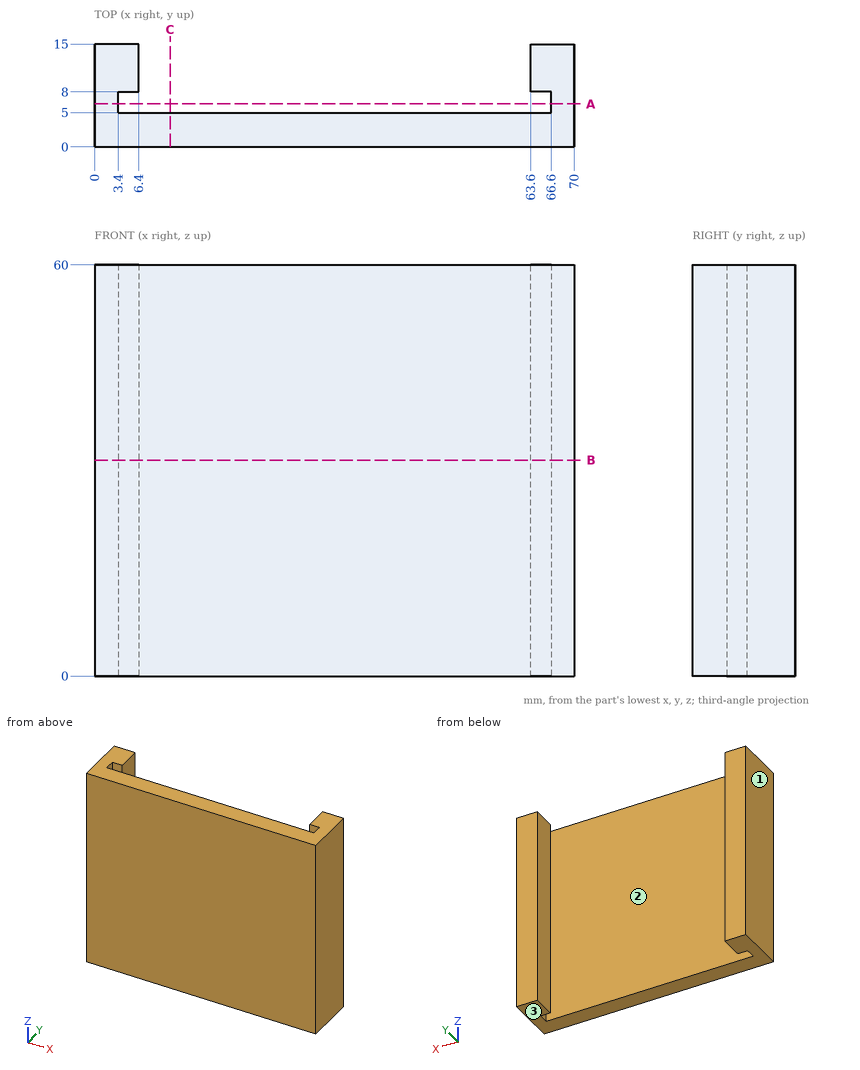
Geometry: see drawing. Coordinates: mm, zero at the bounding-box minimum. Give positions to 0.01 mm unless a question says otherwise; leave off trailing zeros. Order: outer loops, then holes, each group sorted by start corner. A loop starts at its lowest first (then second) coordinate and runs counter-clockwise, first axis right, second up. Notation, with made-up numbers: (17, -21) -> (65, -21) arc R25 cw to (65, 5) -> close; hole circle Ø8 at (55.5, -14.75). An arc over 180 degrees is marked (long way). Write item = value, one per line.
Q1. Pull-direction query (X, two-part tool) for the marked faces 1, 2 and 3; classes: released by +X, released by -X, zero draft, split by the parting line, or undercut.
Data:
face_1 = released by -X
face_2 = undercut
face_3 = zero draft
Q2. Cut plane C-C, the plane x = 11. Output: boundary loops of the cut face in (y, z).
Data:
outline = (0, 0) -> (5, 0) -> (5, 60) -> (0, 60) -> close
Q3. Pin query (flat end, axial travel): pin 1 (3 mm diameter, centred on x = 31, z = 22, fed in from +Y); pin 2 (1 mm diameter, centred on x = 31.5, y = 6, fed in from -Z) (3 decimals). Return the tip coordinate at first contact, or that it passes through.
Data:
pin_1 = 5
pin_2 = through
Q4. Cut plane A-A, the plane y = 6.25. Output: boundary loops of the cut face in (x, z), and give its area (3 significant figures).
Data:
outline = (0, 0) -> (3.4, 0) -> (3.4, 60) -> (0, 60) -> close; (66.6, 0) -> (70, 0) -> (70, 60) -> (66.6, 60) -> close
area = 408 mm^2
Q5. Material intervals for line 1 (X direction, y = 12, z = 27.5); line 2 (X direction, y = 7.75, z = 13.5); line 3 (Y direction, x = 5, z = 31), sorted ascending. Write a range as from..to.
Data:
line_1 = 0..6.4, 63.6..70
line_2 = 0..3.4, 66.6..70
line_3 = 0..5, 8..15
Q6. Cut plane B-B, the plane z = 31.5. Output: boundary loops of the cut face in (x, y).
Data:
outline = (0, 0) -> (70, 0) -> (70, 15) -> (63.6, 15) -> (63.6, 8) -> (66.6, 8) -> (66.6, 5) -> (3.4, 5) -> (3.4, 8) -> (6.4, 8) -> (6.4, 15) -> (0, 15) -> close
